Source: CAD feature listing. Evaluate the final solid. Frame: model axes, mm. A direction names the side the tool comes from. Coordinates: 2 decimals unless noted, no trailing zeros. Order: outer loops, then holes, each group sorted by start corner. A loop starts at its lowest first (then second) coordinate and runs counter-clockwise, first axis right, second up. Notation, with made-up numbers: (-21, 64.25) - (24, 64.25) arc R19 ccw to (24, 87.25) - close; hole circle Ø4 at (83, 44). An arc over 180 degrees is marked (long way). One line per question, with ' | ' between items. Start each with the question number.
(1) Section D-D (x = -45.25). Return the cut outline in (y, z).
(2) Draft query along Y for faces 5 (the cylindrical face through (-38.65, 18.4, -0.63)), 6 (the flat face through (-48.251, 39, -1)), 7 (the flat face through (-48.944, 22.112, -0.626)). Return one class per face: +Y half, -Y half, draft (parallel to the pull), parting line (faces both ways), or undercut.
(3) Access query for faces 1 (the flat face through (-41.278, 25.967, -0.626)), 2 (the flat face through (-47.57, 23, -0.63)), 3 (the flat face through (-33.636, 27.455, -0.626)), 4 (the flat face through (-44.65, 9, -1)). Directions: +Z, -Z, +X, -X, +Y, -Y. A direction counts if a zero-diameter tool reaches every point of the face in a straight line with its end or side. Return the directions, or none.
(4) Section B-B (x = -40). Return the cut outline in (y, z).
(5) Section C-C (y = 30.5). Return the cut outline in (x, z).
(6) Section A-A (z = -0.4). Return the cut outline in (x, y), then the cut area to 3 significant figures.
(7) Contact query for flat-ended pins moving along their axis: P1, Ø0.6, axis at y = 39, z = -0.5, coming from the -X side; P2, Ø8, axis at x = -43, y = 28.5, coming from the +Z side. Output: stop coordinate, or through.
(8) Line query: line 1 along Y through (x, z) = (-38.75, -0.45); line 2 along X through (y, z) = (23, -0.9); line 3 along Y through (x, z) = (-40.5, -0.1). Output: solid intervals per line, ascending.
from build123d import *

# Parameters (mm, degrees)
F1_DEPTH = 1.27


with BuildPart() as f1:
    # F0 (on Top) → F1 (new body)
    with BuildSketch(Plane.XY):
        with BuildLine():
            Line((-44.650044, 11.810658), (-42.345528, 8.785976))
            ThreePointArc((-42.345528, 8.785976), (-36.013085, 16.14737), (-34.54626, 25.746243))
            ThreePointArc((-34.54626, 25.746243), (-34.705251, 26.752672), (-34.922194, 27.748218))
            ThreePointArc((-34.922194, 27.748218), (-39.059576, 35.431946), (-46.378434, 40.185042))
            Line((-46.378434, 40.185042), (-48.250854, 36.728263))
            ThreePointArc((-48.250854, 36.728263), (-47.262902, 36.481943), (-46.296505, 36.161318))
            ThreePointArc((-46.296505, 36.161318), (-40.861402, 32.378631), (-37.901269, 26.455229))
            ThreePointArc((-37.901269, 26.455229), (-37.849542, 26.205506), (-37.802577, 25.954845))
            ThreePointArc((-37.802577, 25.954845), (-37.766593, 25.742227), (-37.734035, 25.529058))
            ThreePointArc((-37.734035, 25.529058), (-37.704911, 25.315392), (-37.67923, 25.101285))
            ThreePointArc((-37.67923, 25.101285), (-38.69112, 18.30755), (-42.936155, 12.907694))
            ThreePointArc((-42.936155, 12.907694), (-43.772245, 12.326595), (-44.650044, 11.810658))
        make_face()
        with BuildLine():
            Line((-46.39398, 23.878697), (-44.650044, 11.810658))
            ThreePointArc((-44.650044, 11.810658), (-43.772245, 12.326595), (-42.936155, 12.907694))
            Line((-42.936155, 12.907694), (-44.554657, 24.107726))
            Line((-44.554657, 24.107726), (-44.61633, 24.534506))
            Line((-44.61633, 24.534506), (-46.488751, 24.534506))
            Line((-46.488751, 24.534506), (-46.39398, 23.878697))
        make_face()
        with BuildLine():
            Line((-46.569266, 25.091674), (-46.488751, 24.534506))
            Line((-46.488751, 24.534506), (-44.61633, 24.534506))
            Line((-44.61633, 24.534506), (-44.678004, 24.961286))
            Line((-44.678004, 24.961286), (-44.750853, 25.465404))
            Line((-44.750853, 25.465404), (-46.296505, 36.161318))
            ThreePointArc((-46.296505, 36.161318), (-47.262902, 36.481943), (-48.250854, 36.728263))
            Line((-48.250854, 36.728263), (-46.569266, 25.091674))
        make_face()
        Polygon((-47.014023, 23.789095), (-46.488751, 24.534506), (-47.228107, 24.996466), (-48.110645, 25.547888), (-49.754124, 25.547888), (-49.754124, 23.612555), (-49.754124, 21.995388), (-48.110645, 22.232885), align=None)
        with BuildLine():
            ThreePointArc((-34.922194, 27.748218), (-34.705251, 26.752672), (-34.54626, 25.746243))
            Line((-34.54626, 25.746243), (-32.386307, 27.169833))
            Line((-32.386307, 27.169833), (-34.922194, 27.748218))
        make_face()
        Polygon((-44.650044, 7.030156), (-42.345528, 8.785976), (-44.650044, 11.810658), align=None)
        Polygon((-48.250854, 36.728263), (-46.378434, 40.185042), (-48.250854, 40.817065), align=None)
        with BuildLine():
            Line((-44.678004, 24.961286), (-37.802577, 25.954845))
            ThreePointArc((-37.802577, 25.954845), (-37.849542, 26.205506), (-37.901269, 26.455229))
            Line((-37.901269, 26.455229), (-44.750853, 25.465404))
            Line((-44.750853, 25.465404), (-44.678004, 24.961286))
        make_face()
        Polygon((-44.61633, 24.534506), (-37.740904, 25.528065), (-37.802577, 25.954845), (-44.678004, 24.961286), align=None)
        Polygon((-47.228107, 24.996466), (-46.488751, 24.534506), (-46.569266, 25.091674), align=None)
        Polygon((-47.014023, 23.789095), (-46.39398, 23.878697), (-46.488751, 24.534506), align=None)
    extrude(amount=-F1_DEPTH)


solid = f1.part
Response values:
1) outline: (15.96, -1.27) - (28.92, -1.27) - (28.92, 0) - (15.96, 0) - close; (35.72, -1.27) - (39.76, -1.27) - (39.76, 0) - (35.72, 0) - close
2) face 5: undercut | face 6: draft | face 7: -Y half
3) face 1: +Z, -Z | face 2: +Z, -Z, -Y | face 3: +Z, -Z, +X, +Y | face 4: +Z, -Z, -X, -Y
4) outline: (10.63, -1.27) - (15.95, -1.27) - (15.95, 0) - (10.63, 0) - close; (25.2, -1.27) - (26.15, -1.27) - (26.15, 0) - (25.2, 0) - close; (31.27, -1.27) - (36.38, -1.27) - (36.38, 0) - (31.27, 0) - close
5) outline: (-47.35, -1.27) - (-45.48, -1.27) - (-45.48, 0) - (-47.35, 0) - close; (-39.5, -1.27) - (-35.85, -1.27) - (-35.85, 0) - (-39.5, 0) - close
6) outline: (-49.75, 22) - (-48.11, 22.23) - (-47.01, 23.79) - (-46.39, 23.88) - (-44.65, 11.81) - (-44.65, 7.03) - (-42.35, 8.79) arc R17.61 ccw to (-34.55, 25.75) - (-32.39, 27.17) - (-34.92, 27.75) arc R17.61 ccw to (-46.38, 40.19) - (-48.25, 40.82) - (-48.25, 36.73) - (-46.57, 25.09) - (-47.23, 25) - (-48.11, 25.55) - (-49.75, 25.55) - close; hole (-46.3, 36.16) - (-44.75, 25.47) - (-37.9, 26.46) arc R13.4 ccw to start; hole (-44.62, 24.53) - (-44.55, 24.11) - (-42.94, 12.91) arc R13.4 ccw to (-37.68, 25.1) arc R13.4 ccw to (-37.73, 25.53) arc R13.4 ccw to (-37.8, 25.95) - (-37.74, 25.53) - close | area: 195 mm²
7) P1: stops at x = -48.25 | P2: stops at z = 0
8) line 1: y = 11.92 to 18.17, 25.38 to 26.33, 29.05 to 35.09 | line 2: x = -49.75 to -47.57, -46.27 to -44.39, -37.61 to -34.41 | line 3: y = 10.18 to 15.28, 25.13 to 26.08, 31.94 to 36.83
